Here's how the part is built. I have some questions about the finished solid (model axes, mm). A direction names the side the tool comes from. Round coordinates to 2 decimals unless told otherwise and drop trailing zeros. Order: outer loops, then holes, each group sorted by start corner. A loop starts at its lowest first (then second) coordinate and runs counter-clockwise, first axis right, second up.
```python
from build123d import *

# Parameters (mm, degrees)
F0_W      = 130
F0_H      = 80
F1_DEPTH  = 65
F4_DEPTH  = 90
F6_D      = 50
F8_R      = 10
F9_DEPTH  = 100
F7_R      = 10
F10_DEPTH = 100


with BuildPart() as f1:
    # F0 (on Front) → F1 (new body)
    with BuildSketch(Plane.XZ):
        with Locations((-3.5409145057, -0.5533536838)):
            Rectangle(F0_W, F0_H)
    extrude(amount=F1_DEPTH)

    # F2: F1 across face


with BuildPart() as f1_1:
    add(f1.part)
    add(f1.part.mirror(Plane(origin=(-3.5409145057, 0, -0.5533536838), x_dir=(1, 0, 0), z_dir=(0, 1, 0))))

    # F3 (on Right) → F4 (join, symmetric)
    with BuildSketch(Plane.YZ):
        with BuildLine():
            Line((32.4888588476, 39.8981455717), (-32.4888588476, 39.8981455717))
            ThreePointArc((-32.4888588476, 39.8981455717), (0, 6.9546503664), (32.4888588476, 39.8981455717))
        make_face()
    extrude(amount=F4_DEPTH, both=True)

    # F6 (through all)
    with Locations(Plane(origin=(-90, 0, 0), x_dir=(0, -1, 0), z_dir=(-1, 0, 0))):
        with Locations((0, 39.8981455717)):
            Hole(F6_D / 2)

    # F8 (on face) → F9 (cut)
    with BuildSketch(Plane.XY.offset(39.4466463162)):
        with Locations((0, 48.0979235456)):
            Circle(F8_R)
    extrude(amount=-F9_DEPTH, mode=Mode.SUBTRACT)

    # F7 (on face) → F10 (cut)
    with BuildSketch(Plane.XY.offset(39.4466463162)):
        with Locations((0, -46.4860715879)):
            Circle(F7_R)
    extrude(amount=-F10_DEPTH, mode=Mode.SUBTRACT)


solid = f1_1.part
```
1. If we mould it in two halves opening along X, with no side actions, what happens to faces 1 (the cylindrical face through (-1.3, -36.57, 0.01)), 2 (the flat face through (-4, -56, 39.447)), 3 (the flat face through (61.459, -1, -10))? For each: released by +X, released by -X, zero draft, split by the parting line, or undercut.
Evaluation:
face 1: undercut
face 2: zero draft
face 3: released by +X
2. If we section it at B-B, the plane z = 27.5: Write out the boundary of the cut face in (x, y), and give its area (3 significant figures).
Evaluation:
outline: (-90, -30.22) - (-68.54, -30.22) - (-68.54, -65) - (61.46, -65) - (61.46, -30.22) - (90, -30.22) - (90, -21.71) - (-90, -21.71) - close; (-90, 21.71) - (90, 21.71) - (90, 30.22) - (61.46, 30.22) - (61.46, 65) - (-68.54, 65) - (-68.54, 30.22) - (-90, 30.22) - close; hole circle Ø20 at (0, -46.49); hole circle Ø20 at (0, 48.1)
area: 11,500 mm2
3. On a 3-axis mill with a long thin cutter (end or side, diameter ignored), from which of +Z, -Z, +X, -X, +Y, -Y can I reach the whole of each face in a straight line? I mean faces 4 (the flat face through (-90, -3, 14)), 5 (the flat face through (-68.541, -1, -10)), 6 (the flat face through (-4, 38, 39.447)). Say none if no direction works.
Evaluation:
face 4: +Z, -Z, -X, +Y, -Y
face 5: -Z, -X
face 6: +Z, +X, -X, +Y
4. If we section it at A-A, the plane x = 0: Write out the boundary of the cut face in (y, z), and give its area (3 significant figures).
Evaluation:
outline: (-65, -40.55) - (-56.49, -40.55) - (-56.49, 39.45) - (-65, 39.45) - close; (-36.49, -40.55) - (38.1, -40.55) - (38.1, 39.45) - (32.49, 39.45) arc R32.49 ccw to (32.49, 39.9) - (25, 39.9) arc R25 cw to (-25, 39.9) - (-32.49, 39.9) arc R32.49 ccw to (-32.49, 39.45) - (-36.49, 39.45) - close; (58.1, -40.55) - (65, -40.55) - (65, 39.45) - (58.1, 39.45) - close
area: 6,250 mm2
5. If we section it at D-D, the plane z = 11.5: Write out the boundary of the cut face in (x, y).
Evaluation:
outline: (-90, -16.57) - (-68.54, -16.57) - (-68.54, -65) - (61.46, -65) - (61.46, -16.57) - (90, -16.57) - (90, 16.57) - (61.46, 16.57) - (61.46, 65) - (-68.54, 65) - (-68.54, 16.57) - (-90, 16.57) - close; hole circle Ø20 at (0, -46.49); hole circle Ø20 at (0, 48.1)
6. I'm going to push flat-ended pins straight in: P1, Ø2, axis at y = 4, z = -31, coming from the -X side; P2, Ø23, axis at x = 0, y = 48.1, coming from the +Z side; P3, Ø12, axis at x = 0, y = -46.49, coming from the -Z side; P4, Ø8, axis at y = 2, z = -6.5, coming from the +X side. Where does each tip first touch, or does it pass through?
Evaluation:
P1: stops at x = -68.54
P2: stops at z = 39.45
P3: passes through
P4: stops at x = 61.46
7. I need wall thicknesses on probe 1 along Y at (x, z) = (0, -19.5); probe 2 along Y at (x, z) = (-8.5, -16.5); probe 3 along X at (y, z) = (6.5, -32.5). Which ranges of each line are inside material? Lowest first, please.
Evaluation:
probe 1: y = -65 to -56.49, -36.49 to 38.1, 58.1 to 65
probe 2: y = -65 to -51.75, -41.22 to 42.83, 53.37 to 65
probe 3: x = -68.54 to 61.46
8. If we section it at C-C, the plane y = 0: Write out the boundary of the cut face in (x, z), and give its area (3 significant figures).
Evaluation:
outline: (-90, 6.95) - (-68.54, 6.95) - (-68.54, -40.55) - (61.46, -40.55) - (61.46, 6.95) - (90, 6.95) - (90, 14.9) - (-90, 14.9) - close
area: 7,610 mm2
